Geometry check sheet. Reference: the model listing, model coordinates, mm. A direction names the side the tool comes from. Coordinates: 2 decimals unless noted, no trailing zeros. Write each loop counter-clockwise with the first axis right and the second up, starting at its lowest first coordinate (ties: lowest second). Pieces come first, ordered by that corner, then holes.
from build123d import *

# Parameters (mm, degrees)
SKETCH2_W                     = 800
SKETCH2_H                     = 53
BASE_FLANGE1_DEPTH            = 3
EDGE_FLANGE1_STRIP_W          = 18
EDGE_FLANGE1_STRIP_H          = 3
EDGE_FLANGE1_STRIP_CUT_DEPTH  = 697
EDGE_FLANGE1_RELIEF_W         = 18.9
EDGE_FLANGE1_RELIEF_H         = 0.9
EDGE_FLANGE1_RELIEF_CUT_DEPTH = 3
EDGE_FLANGE1_DEPTH            = 697
EDGE_FLANGE1_FLAT_DEPTH       = 3
EDGE_FLANGE2_STRIP_W          = 18
EDGE_FLANGE2_STRIP_H          = 3
EDGE_FLANGE2_STRIP_CUT_DEPTH  = 694
EDGE_FLANGE2_DEPTH            = 694
EDGE_FLANGE3_STRIP_W          = 18
EDGE_FLANGE3_STRIP_H          = 3
EDGE_FLANGE3_STRIP_CUT_DEPTH  = 694
EDGE_FLANGE3_DEPTH            = 694
FILLET1_R                     = 10
CUT_EXTRUDE2_DEPTH            = 3
LPATTERN1_COUNT               = 4
LPATTERN1_PITCH               = 195.333333333
SKETCH20_R                    = 6
CUT_EXTRUDE3_DEPTH            = 3
SKETCH21_R                    = 6
CUT_EXTRUDE4_DEPTH            = 3
LPATTERN2_COUNT               = 5
LPATTERN2_PITCH               = 141.25
SKETCH22_R                    = 2
CUT_EXTRUDE5_DEPTH            = 3
LPATTERN3_COUNT               = 4
LPATTERN3_PITCH               = 218


# Sheet-metal steps are written as plain solids
with BuildPart() as part:
    # Sketch2 → Base-Flange1 (new body)
    with BuildSketch(Plane.XY):
        Rectangle(SKETCH2_W, SKETCH2_H)
    extrude(amount=-BASE_FLANGE1_DEPTH)

    # Edge-Flange1 strip (across the edge) → Edge-Flange1 strip cut (cut)
    with BuildSketch(Plane(origin=(348.5, -26.5, -3), x_dir=(0, 1, 0), z_dir=(-1, 0, 0))):
        with Locations((-3, -1.5)):
            Rectangle(EDGE_FLANGE1_STRIP_W, EDGE_FLANGE1_STRIP_H)
    extrude(amount=EDGE_FLANGE1_STRIP_CUT_DEPTH, mode=Mode.SUBTRACT)

    # Edge-Flange1 relief (on the sheet) → Edge-Flange1 relief cut (cut)
    with BuildSketch(Plane(origin=(348.5, -20.5, -3), x_dir=(0, 1, 0), z_dir=(0, 0, -1))):
        with Locations((-8.55, 0.45)):
            Rectangle(EDGE_FLANGE1_RELIEF_W, EDGE_FLANGE1_RELIEF_H)
        with Locations((-8.55, -697.45)):
            Rectangle(EDGE_FLANGE1_RELIEF_W, EDGE_FLANGE1_RELIEF_H)
    extrude(amount=-EDGE_FLANGE1_RELIEF_CUT_DEPTH, mode=Mode.SUBTRACT)

    # Edge-Flange1 bend section (across the edge) → Edge-Flange1 (add)
    with BuildSketch(Plane(origin=(348.5, -26.5, -3), x_dir=(0, 1, 0), z_dir=(-1, 0, 0))):
        with BuildLine():
            Line((0, 3), (3, 3))
            ThreePointArc((3, 3), (3.878679656, 0.878679656), (6, 0))
            Line((6, 0), (6, -3))
            ThreePointArc((6, -3), (1.757359313, -1.242640687), (0, 3))
        make_face()
    extrude(amount=EDGE_FLANGE1_DEPTH)

    # Edge-Flange1 profile (on flange) → Edge-Flange1 flat (add)
    with BuildSketch(Plane(origin=(0, -26.5, -3), x_dir=(1, 0, 0), z_dir=(0, 1, 0))):
        Polygon((-348.5, 16.5), (-348.5, 3), (348.5, 3), (348.5, 16.5), (347, 16.5), (347, 37.5), (348.5, 37.5), (348.5, 116.5), (347, 116.5), (347, 137.5), (348.5, 137.5), (348.5, 147.5), (347, 147.5), (347, 157), (-347, 157), (-347, 147.5), (-348.5, 147.5), (-348.5, 137.5), (-347, 137.5), (-347, 116.5), (-348.5, 116.5), (-348.5, 37.5), (-347, 37.5), (-347, 16.5), align=None)
    extrude(amount=EDGE_FLANGE1_FLAT_DEPTH)

    # Edge-Flange2 strip (across the edge) → Edge-Flange2 strip cut (cut)
    with BuildSketch(Plane(origin=(-347, -26.5, -160), x_dir=(0, 0, 1), z_dir=(1, 0, 0))):
        with Locations((-3, -1.5)):
            Rectangle(EDGE_FLANGE2_STRIP_W, EDGE_FLANGE2_STRIP_H)
    extrude(amount=EDGE_FLANGE2_STRIP_CUT_DEPTH, mode=Mode.SUBTRACT)

    # Edge-Flange2 section (across the edge) → Edge-Flange2 (add)
    with BuildSketch(Plane(origin=(-347, -26.5, -160), x_dir=(0, 0, 1), z_dir=(1, 0, 0))):
        with BuildLine():
            Line((0, 3), (0, 33))
            Line((0, 33), (3, 33))
            Line((3, 33), (3, 3))
            ThreePointArc((3, 3), (3.878679656, 0.878679656), (6, 0))
            Line((6, 0), (6, -3))
            ThreePointArc((6, -3), (1.757359313, -1.242640687), (0, 3))
        make_face()
    extrude(amount=EDGE_FLANGE2_DEPTH)

    # Edge-Flange3 strip (across the edge) → Edge-Flange3 strip cut (cut)
    with BuildSketch(Plane(origin=(-347, -59.5, -157), x_dir=(0, 1, 0), z_dir=(1, 0, 0))):
        with Locations((-3, -1.5)):
            Rectangle(EDGE_FLANGE3_STRIP_W, EDGE_FLANGE3_STRIP_H)
    extrude(amount=EDGE_FLANGE3_STRIP_CUT_DEPTH, mode=Mode.SUBTRACT)

    # Edge-Flange3 section (across the edge) → Edge-Flange3 (add)
    with BuildSketch(Plane(origin=(-347, -59.5, -157), x_dir=(0, 1, 0), z_dir=(1, 0, 0))):
        with BuildLine():
            Line((0, 3), (0, 23))
            Line((0, 23), (3, 23))
            Line((3, 23), (3, 3))
            ThreePointArc((3, 3), (3.878679656, 0.878679656), (6, 0))
            Line((6, 0), (6, -3))
            ThreePointArc((6, -3), (1.757359313, -1.242640687), (0, 3))
        make_face()
    extrude(amount=EDGE_FLANGE3_DEPTH)

    # Fillet1
    fillet1_edges = [part.edges().sort_by_distance(p)[0] for p in [
        (-400, 26.5, -1.5),
        (400, 26.5, -1.5),
    ]]
    fillet(fillet1_edges, radius=FILLET1_R)

    # Sketch19 → Cut-Extrude2 (cut)
    with BuildSketch(Plane(origin=(0, 0, -160), x_dir=(-1, 0, 0), z_dir=(0, 0, -1))):
        Polygon((-286.591412012, -39.5), (-289.795706006, -33.95), (-296.204293994, -33.95), (-299.408587988, -39.5), (-296.204293994, -45.05), (-289.795706006, -45.05), align=None)
    cut_extrude2 = extrude(amount=-CUT_EXTRUDE2_DEPTH, mode=Mode.SUBTRACT)

    # LPattern1: Cut-Extrude2 ×4
    with Locations(*[(-i * LPATTERN1_PITCH, 0, 0) for i in range(1, LPATTERN1_COUNT)]):
        add(cut_extrude2, mode=Mode.SUBTRACT)

    # Sketch20 → Cut-Extrude3 (cut)
    with BuildSketch(Plane(origin=(0, 0, -3), x_dir=(-1, 0, 0), z_dir=(0, 0, -1))):
        with Locations((-380, 6.5)):
            Circle(SKETCH20_R)
        with Locations((380, 6.5)):
            Circle(SKETCH20_R)
    extrude(amount=-CUT_EXTRUDE3_DEPTH, mode=Mode.SUBTRACT)

    # Sketch21 → Cut-Extrude4 (cut)
    with BuildSketch(Plane(origin=(0, 0, -3), x_dir=(-1, 0, 0), z_dir=(0, 0, -1))):
        with Locations((-282.5, 6.5)):
            Circle(SKETCH21_R)
    cut_extrude4 = extrude(amount=-CUT_EXTRUDE4_DEPTH, mode=Mode.SUBTRACT)

    # LPattern2: Cut-Extrude4 ×5
    with Locations(*[(-i * LPATTERN2_PITCH, 0, 0) for i in range(1, LPATTERN2_COUNT)]):
        add(cut_extrude4, mode=Mode.SUBTRACT)

    # Sketch22 → Cut-Extrude5 (cut)
    with BuildSketch(Plane(origin=(0, -23.5, 0), x_dir=(1, 0, 0), z_dir=(0, 1, 0))):
        with Locations(Location((-327, 16, 0), (0, 0, 270))):
            Circle(SKETCH22_R)
        with Locations(Location((-327, 39, 0), (0, 0, 270))):
            Circle(SKETCH22_R)
        with Locations(Location((-327, 125, 0), (0, 0, 270))):
            Circle(SKETCH22_R)
    cut_extrude5 = extrude(amount=-CUT_EXTRUDE5_DEPTH, mode=Mode.SUBTRACT)

    # LPattern3: Cut-Extrude5 ×4
    with Locations(*[(i * LPATTERN3_PITCH, 0, 0) for i in range(1, LPATTERN3_COUNT)]):
        add(cut_extrude5, mode=Mode.SUBTRACT)


solid = part.part
1. Draft check along Y on faces 4 (the flat face through (-5, -42, -157)), 5 (the flat face through (-347, -45, -158)), 6 (the flat face through (-5, -59.5, -144)). Enter one of: released by +Y, released by -Y, zero draft, split by the parting line, or undercut.
Computed values:
face 4: undercut
face 5: zero draft
face 6: released by -Y
2. Sectioned sample at A-A, the plane x = 258.5. Record the boundary of the cut face in (y, z), and give its area (3 significant figures).
Computed values:
outline: (-59.5, -154) arc R6 ccw to (-53.5, -160) - (-29.5, -160) arc R6 ccw to (-23.5, -154) - (-23.5, -6) arc R3 cw to (-20.5, -3) - (26.5, -3) - (26.5, 0) - (-20.5, 0) arc R6 ccw to (-26.5, -6) - (-26.5, -154) arc R3 cw to (-29.5, -157) - (-53.5, -157) arc R3 cw to (-56.5, -154) - (-56.5, -134) - (-59.5, -134) - close
area: 781 mm2
3. Thickness scan on line 1 along X through (y, z) = (-24.75, -16); line 2 along X through (y, z) = (-24, -39); line 3 along Z through (x, y) = (-166, -14.5). Record the ranges inside material, lowest first.
Computed values:
line 1: x = -348.5 to -329, -325 to -111, -107 to 107, 111 to 325, 329 to 348.5
line 2: x = -347 to -329, -325 to -111, -107 to 107, 111 to 325, 329 to 347
line 3: z = -3 to 0
4. Sectioned sample at B-B, the plane z = -67.5. Record the boundary of the cut face in (x, y).
Computed values:
outline: (-348.5, -26.5) - (348.5, -26.5) - (348.5, -23.5) - (-348.5, -23.5) - close
5. Gauge pin test, flat ends, axial feed: pin 1 Ø6.5 at (x, z) = (109, -125) entering from -Y; pin 2 Ø2 at (x, y) = (263.5, -31.5) entering from +Z; pin 3 Ø1.5 at (y, z) = (-25, -29) entering from +X; pin 4 Ø3 at (x, z) = (327, -125) entering from +Y. Record the tip position at first contact, or that the pin passes through.
Computed values:
pin 1: stops at y = -26.5
pin 2: stops at z = -157
pin 3: stops at x = 347
pin 4: passes through
6. Access from +Z, -Z, +X, -X, +Y, -Y to the whole of each face (thin tool, end or side, straight path). Record for faces 1 (the flat face through (-5, -23.5, -81)), 2 (the flat face through (-5, -56.5, -144)), 3 (the flat face through (-6, 0, 0)).
Computed values:
face 1: -Z, +X, -X, +Y
face 2: +Z, +X, -X
face 3: +Z, +X, -X, +Y, -Y
7. Sectioned sample at C-C, the plane y = -11.5. Record the boundary of the cut face in (x, z), and give its area (3 significant figures).
Computed values:
outline: (-400, -3) - (400, -3) - (400, 0) - (-400, 0) - close
area: 2,400 mm2
